Here's how the part is built. I have some questions about the finished solid (model axes, mm). Coordinates: 2 decimals unless noted, no trailing zeros. Loops run counter-clockwise (first coordinate to the right, second up) from the corner with the lowest first, then second, coordinate; pieces in that order, holes last. Notation, with made-up numbers: (-32.75, -32) - (4.25, -32) arc R28 ccw to (4.25, 2) - close; hole circle Ø3 at (68, 47). An arc over 180 degrees is marked (long way). Use a Markdown table: item, result.
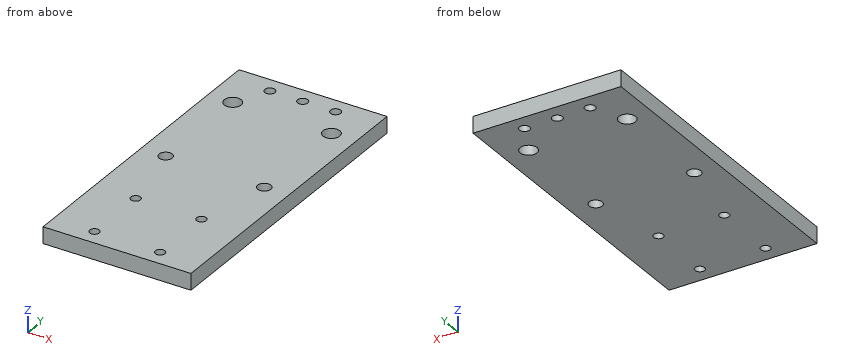
Autodesk Inventor part; units mm, degrees
ref_plane "YZ Plane" through (0, 0, 0) normal (1, 0, 0) x (0, 1, 0)
ref_plane "XZ Plane" through (0, 0, 0) normal (0, 1, 0) x (-1, 0, 0)
ref_plane "XY Plane" through (0, 0, 0) normal (0, 0, 1) x (1, 0, 0)
sketch "Sketch1" plane through (0, 0, 0) normal (0, 0, 1) x (1, 0, 0)
  line L0 (-19.05, 0) -> (19.05, 0) construction
  circle A0 centre (-19.05, 0) radius 3.2639
  circle A1 centre (19.05, 0) radius 3.2639
  line L1 (-28.575, 19.5947) -> (-28.575, -101.6)
  line L2 (-28.575, -101.6) -> (28.575, -101.6)
  line L3 (28.575, -101.6) -> (28.575, 19.5947)
  line L4 (-26.7151, 24.0849) -> (-4.4901, 46.3099)
  line L5 (4.4901, 46.3099) -> (26.7151, 24.0849)
  arc A2 (4.4901, 46.3099) -> (-4.4901, 46.3099) centre (0, 41.8197) ccw
  arc A3 (-26.7151, 24.0849) -> (-28.575, 19.5947) centre (-22.225, 19.5947) ccw
  arc A4 (28.575, 19.5947) -> (26.7151, 24.0849) centre (22.225, 19.5947) ccw
  line L6 (-28.575, 19.05) -> (28.575, 19.05)
  line L7 (-12.7, 12.7) -> (12.7, 12.7) construction
  line L8 (-12.7, -69.85) -> (12.7, -69.85) construction
  point P0 (0, 0)
  point P1 (0, 0)
  point P2 (0, 50.8)
  point P3 (28.575, 22.225)
  point P4 (-28.575, 22.225)
  point P5 (0, -101.6)
  point P6 (0, 12.7)
  point P7 (0, 12.7)
  point P8 (-12.7, -95.25)
  point P9 (12.7, -95.25)
  point P10 (0, -69.85)
  dimension "d0" = 6.5278
  dimension "d1" = 38.1
  dimension "d4" = 101.6
  dimension "d17" = 152.4
  dimension "d18" = 57.15
  dimension "d19" = 6.35
  dimension "d20" = 120.65
  dimension "d21" = 25.4
  dimension "d29" = 6.35
  dimension "d32" = 25.4
  dimension "d33" = 25.4
  dimension "d34" = 6.35
extrude "Extrusion1" add sketch "Sketch1" along normal blind 6.35 contours L6 L3 L2 L1
sketch "Sketch2" plane through (0, 0, 6.35) normal (0, 0, 1) x (1, 0, 0)
  line L0 (-19.05, -41.275) -> (19.05, -41.275) construction
  line L1 (-28.575, -101.6) -> (28.575, -101.6)
  point P0 (0, 0)
  point P1 (0, -41.275)
  dimension "d8" = 38.1
  dimension "d9" = 60.325
hole "Hole1" at (-19.05, -41.275, 6.35) at (19.05, -41.275, 6.35) direction (0, 0, -1) diameter 5.1054 end through all
hole "Hole2" at (-12.7, 12.7, 0) at (0, 12.7, 0) at (12.7, 12.7, 0) direction (0, 0, 1) diameter 3.9624 end through all
hole "Hole3" at (-12.7, -69.85, 0) at (12.7, -69.85, 0) at (-12.7, -95.25, 0) at (12.7, -95.25, 0) direction (0, 0, 1) diameter 3.683 end through all
properties part number "CL7-005aa" material "Aluminum 6061"
Q1. Will this pin go through, and if not, where does the flat tip stop? P1, Ø3, axis at x = 12.7, y = -95.25, coming from the +Z side.
Check values:
| item | result |
|---|---|
| P1 | through |
Q2. I want a section at B-B, the plane x = -19.05. Write out the boundary of the cut face in (y, z), then the cut area to 3 significant figures.
Check values:
| item | result |
|---|---|
| outline | (-101.6, 0) - (-43.83, 0) - (-43.83, 6.35) - (-101.6, 6.35) - close; (-38.72, 0) - (-3.26, 0) - (-3.26, 6.35) - (-38.72, 6.35) - close; (3.26, 0) - (19.05, 0) - (19.05, 6.35) - (3.26, 6.35) - close |
| area | 692 mm^2 |
Q3. Please list where these lines run through material, in increasing order: L1, parallel to Y at x = 13, z = 6.25; L2, parallel to X at y = -95.25, z = 4.5 (1 decimal); L3, parallel to X at y = -70.5, z = 4.75 (3 decimals). Write a range as from..to.
Check values:
| item | result |
|---|---|
| L1 | -101.6..-97.07, -93.43..-71.67, -68.03..10.74, 14.66..19.05 |
| L2 | -28.6..-14.5, -10.9..10.9, 14.5..28.6 |
| L3 | -28.575..-14.423, -10.977..10.977, 14.423..28.575 |
Q4. I want a section at C-C, the plane y = -95.25. Give the number of separate pieces and of enclosed holes in the cut face, then the cut area to 3 significant figures.
Check values:
| item | result |
|---|---|
| separate pieces | 3 |
| enclosed holes | 0 |
| area | 316 mm^2 |
Q5. I want a section at D-D, the plane x = -12.7. Write out the boundary of the cut face in (y, z).
Check values:
| item | result |
|---|---|
| outline | (-101.6, 0) - (-97.09, 0) - (-97.09, 6.35) - (-101.6, 6.35) - close; (-93.41, 0) - (-71.69, 0) - (-71.69, 6.35) - (-93.41, 6.35) - close; (-68.01, 0) - (10.72, 0) - (10.72, 6.35) - (-68.01, 6.35) - close; (14.68, 0) - (19.05, 0) - (19.05, 6.35) - (14.68, 6.35) - close |
Q6. I want a section at A-A, the plane y = 12.7. Write out the boundary of the cut face in (x, z) (3 decimals).
Check values:
| item | result |
|---|---|
| outline | (-28.575, 0) - (-14.681, 0) - (-14.681, 6.35) - (-28.575, 6.35) - close; (-10.719, 0) - (-1.981, 0) - (-1.981, 6.35) - (-10.719, 6.35) - close; (1.981, 0) - (10.719, 0) - (10.719, 6.35) - (1.981, 6.35) - close; (14.681, 0) - (28.575, 0) - (28.575, 6.35) - (14.681, 6.35) - close |
